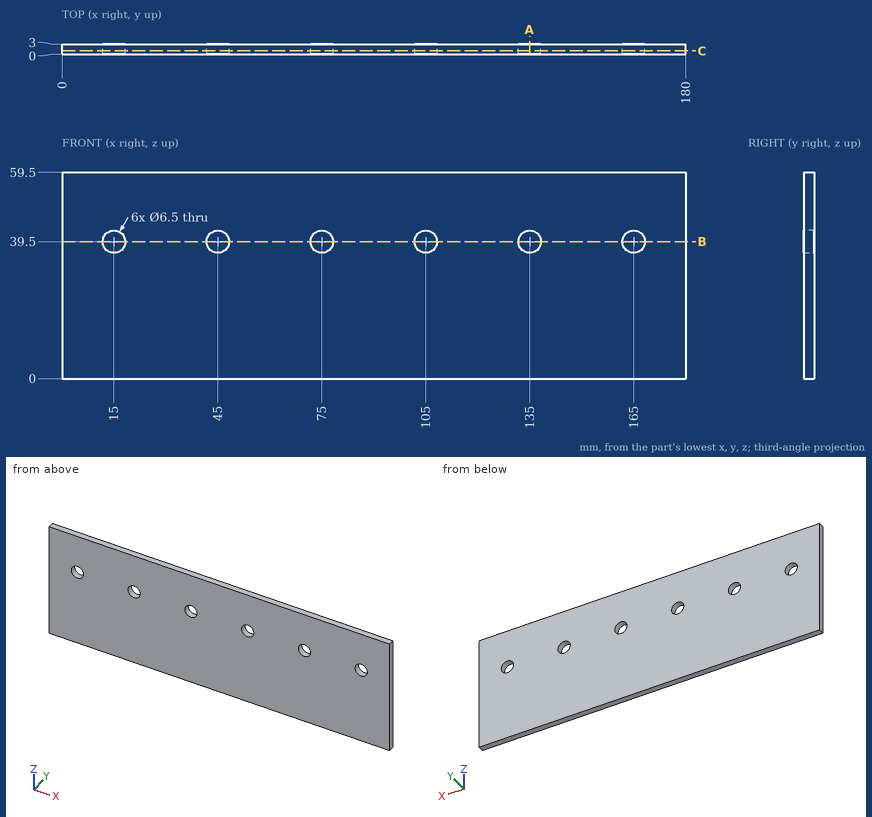
Here's the drawing with two shaded views (mm, measured from the low corner). I have some questions. Give positions to 0.01 mm unless a question says otherwise; leave off trailing zeros. Loops run counter-clockwise (first coordinate to the right, second up) from the corner with the lowest first, then second, coordinate; pieces in that order, holes last. Notation, with made-up numbers: (16.25, 19.25) -> (28.25, 19.25) arc R30 cw to (28.25, 58.25) -> close; hole circle Ø3 at (20.25, 25.25). An arc over 180 degrees is marked (long way). Answer as a JSON object with one key per item and string values. Group by question number.
Item 1: Will this pin go through, and if not, where does the flat tip stop? pin 1 (5 mm diameter, centred on x = 45, z = 39.5, fed in from +Y).
Item 2: Imagine slicing it at B-B on z = 39.5. Write out the boundary of the cut face in (x, y).
Item 3: I need wall thicknesses on L1, parallel to Z at x = 135, y = 1.3. Which ranges of the line are inside material? Lowest first, please.
Item 4: Imagine slicing it at C-C on y = 1.05. Write out the boundary of the cut face in (x, z).
Item 5: Imagine slicing it at A-A on x = 135. Write out the boundary of the cut face in (y, z), then the cut area to 3 significant figures.
Answer list:
{
 "1": {"pin 1": "passes through"},
 "2": {"outline": "(0, 0) -> (11.75, 0) -> (11.75, 3) -> (0, 3) -> close; (18.25, 0) -> (41.75, 0) -> (41.75, 3) -> (18.25, 3) -> close; (48.25, 0) -> (71.75, 0) -> (71.75, 3) -> (48.25, 3) -> close; (78.25, 0) -> (101.75, 0) -> (101.75, 3) -> (78.25, 3) -> close; (108.25, 0) -> (131.75, 0) -> (131.75, 3) -> (108.25, 3) -> close; (138.25, 0) -> (161.75, 0) -> (161.75, 3) -> (138.25, 3) -> close; (168.25, 0) -> (180, 0) -> (180, 3) -> (168.25, 3) -> close"},
 "3": {"L1": "z = 0 to 36.25, 42.75 to 59.5"},
 "4": {"outline": "(0, 0) -> (180, 0) -> (180, 59.5) -> (0, 59.5) -> close; hole circle Ø6.5 at (15, 39.5); hole circle Ø6.5 at (45, 39.5); hole circle Ø6.5 at (75, 39.5); hole circle Ø6.5 at (105, 39.5); hole circle Ø6.5 at (135, 39.5); hole circle Ø6.5 at (165, 39.5)"},
 "5": {"outline": "(0, 0) -> (3, 0) -> (3, 36.25) -> (0, 36.25) -> close; (0, 42.75) -> (3, 42.75) -> (3, 59.5) -> (0, 59.5) -> close", "area": "159 mm2"}
}
